from build123d import *

# Parameters (mm, degrees)
F0_W     = 196.9244256616
F0_H     = 103.4533828497
F1_DEPTH = 101.6
F2_W     = 103.0500568449
F2_H     = 91.7569026351
F3_DEPTH = 103.4543828497
F4_R     = 17.5216087131
F5_DEPTH = 196.9254256616
F6_W     = 189.05954808
F6_H     = 94.9835181236
F7_DEPTH = 52.3746936212
F8_W     = 189.05954808
F8_H     = 94.9835181236
F9_DEPTH = 49.2273063788


with BuildPart() as f1:
    # F0 (on Top) → F1 (new body)
    with BuildSketch(Plane.XY):
        with Locations((0.1512430608, -5.2936673164)):
            Rectangle(F0_W, F0_H)
    extrude(amount=F1_DEPTH)

    # F2 (on face) → F3 (cut, through all)
    with BuildSketch(Plane.XZ.offset(57.0203587413)):
        with Locations((3.3274423331, 95.1047576964)):
            Rectangle(F2_W, F2_H)
    extrude(amount=-F3_DEPTH, mode=Mode.SUBTRACT)

    # F4 (on face) → F5 (cut, through all)
    with BuildSketch(Plane(origin=(-98.31096977, 0, 0), x_dir=(0, -1, 0), z_dir=(-1, 0, 0))):
        with Locations((5.9994906187, 72.1655264497)):
            Circle(F4_R)
    extrude(amount=-F5_DEPTH, mode=Mode.SUBTRACT)

    # F6 (on face) → F7 (cut, through all)
    with BuildSketch(Plane.XY.offset(49.2263063788)):
        with Locations((-0.3025047481, -4.9911737442)):
            Rectangle(F6_W, F6_H)
    extrude(amount=F7_DEPTH, mode=Mode.SUBTRACT)

    # F8 (on face) → F9 (cut, through all)
    with BuildSketch(Plane.XY.offset(49.2263063788)):
        with Locations((-0.3025047481, -4.9911737442)):
            Rectangle(F8_W, F8_H)
    extrude(amount=-F9_DEPTH, mode=Mode.SUBTRACT)


solid = f1.part
Source: CAD feature listing. Evaluate the final solid. Frame: model axes, mm. A direction names the side the tool comes from. Round coordinates to 2 decimals unless told otherwise and drop trailing zeros. Write each loop counter-clockwise with the first axis right and the second up, starting at its lowest first coordinate (ties: lowest second). Pieces come first, ordered by that corner, then holes. Notation, with made-up numbers: (-38, -15) - (-8, -15) arc R10 cw to (-8, -6) - close; hole circle Ø7 at (44.5, 40.5). An arc over 180 degrees is marked (long way). Use CSV: the item, a comma, the result in double quotes. Start each with the question number.
(1) Cut plane D-D, the plane z = 45. Return loops of the section in (x, y), and give its area (3 significant figures).
(2) First-contact query: pin 1 Ø3.5 at (x, y) = (24, -55) entering from +Z. Flat tip, straight axial feed; report the tip coordinate or a pass-through.
(3) Cut plane B-B, the plane y = -33. Return loops of the section in (x, z).
(4) Cut plane C-C, the plane z = 65.5. Return loops of the section in (x, y), and give its area (3 significant figures).
(5) Cut plane A-A, the plane x = 66. Return loops of the section in (y, z).
(6) Set-up query: faces 1 (the face through (54.852, -55, 75)), 2 (the face through (98.613, -6, 50)), 3 (the face through (-2, -52.483, 40)). Return all of +Z, -Z, +X, -X, +Y, -Y with unobstructed straight access to the full face (end or side cutting, diameter ignored); none if empty.
(7) Material intervals for probe 1 along X at (y, z) = (0, 10); probe 2 along Y at (x, z) = (37.5, 37.5), sorted ascending. Write a range as [from, to].
(8) Mould query, pull axis Z, two halves, no side actions, for faces 4 (the face through (-96.6, -2.2, 55.06)), 5 (the face through (54.852, 44, 75)), 6 (the face through (3, -55, 49.226)). Classes: pulls with the +Z half, pulls with the -Z half, needs draft (parallel to the pull), parting line crosses it, or undercut.
Geometry says:
1,outline,"(-98.31, -57.02) - (98.61, -57.02) - (98.61, 46.43) - (-98.31, 46.43) - close; hole (-94.83, -52.48) - (94.23, -52.48) - (94.23, 42.5) - (-94.83, 42.5) - close"
1,area,"2,410 mm²"
2,pin 1,"z = 49.23"
3,outline,"(-98.31, 0) - (-94.83, 0) - (-94.83, 101.6) - (-98.31, 101.6) - close; (94.23, 0) - (98.61, 0) - (98.61, 101.6) - (94.23, 101.6) - close"
4,outline,"(-98.31, -57.02) - (-48.2, -57.02) - (-48.2, -52.48) - (-94.83, -52.48) - (-94.83, -22.2) - (-98.31, -22.2) - close; (-98.31, 10.2) - (-94.83, 10.2) - (-94.83, 42.5) - (-48.2, 42.5) - (-48.2, 46.43) - (-98.31, 46.43) - close; (54.85, -57.02) - (98.61, -57.02) - (98.61, -22.2) - (94.23, -22.2) - (94.23, -52.48) - (54.85, -52.48) - close; (54.85, 42.5) - (94.23, 42.5) - (94.23, 10.2) - (98.61, 10.2) - (98.61, 46.43) - (54.85, 46.43) - close"
4,area,"1,290 mm²"
5,outline,"(-57.02, 0) - (-52.48, 0) - (-52.48, 101.6) - (-57.02, 101.6) - close; (42.5, 0) - (46.43, 0) - (46.43, 101.6) - (42.5, 101.6) - close"
6,face 1,"+Z, +Y, -Y"
6,face 2,"+Z, -Z, +X, +Y, -Y"
6,face 3,"+Z, -Z"
7,probe 1,"[-98.31, -94.83], [94.23, 98.61]"
7,probe 2,"[-57.02, -52.48], [42.5, 46.43]"
8,face 4,"undercut"
8,face 5,"needs draft"
8,face 6,"pulls with the +Z half"
